```python
from build123d import *

# Parameters (mm, degrees)
SKETCH3_R                 = 2.75
BOSS_EXTRUDE3_DEPTH       = 4.5
FILLET13_R                = 15
FILLET14_START            = -4.5
FILLET14_DEPTH            = 9
SKETCH6_W                 = 69.28510074
SKETCH6_H                 = 3
CUT_EXTRUDE3_DEPTH        = 8
F_3_0MM_DOWEL_HOLE1_D     = 4
F_3_0MM_DOWEL_HOLE1_DEPTH = 9
F_3_0MM_DOWEL_HOLE1_TIP   = 1.201721238
CUT_EXTRUDE4_DEPTH        = 9
FILLET16_R                = 3
FILLET17_R                = 10
FILLET18_R                = 1.5


with BuildPart() as part:
    # Sketch3 → Boss-Extrude3 (new, symmetric)
    with BuildSketch(Plane.XY):
        with BuildLine():
            Line((0, 4), (-57, 43))
            Line((-57, 43), (-118.915266557, 43))
            ThreePointArc((-118.915266557, 43), (-123.007557158, 46.323583072), (-128.27688576, 46.488576653))
            Line((-128.27688576, 46.488576653), (-132.896667749, 45.573835187))
            ThreePointArc((-132.896667749, 45.573835187), (-135.482170861, 44.646108184), (-137.681223291, 43))
            Line((-137.681223291, 43), (-192, 43))
            Line((-192, 43), (-192, 30))
            Line((-192, 30), (-137.769349371, 30))
            Line((-137.769349371, 30), (-136.290115263, 28.079175362))
            ThreePointArc((-136.290115263, 28.079175362), (-129.185667244, 24.063000847), (-122.139231824, 28.180109937))
            Line((-122.139231824, 28.180109937), (-121.157209597, 30))
            Line((-121.157209597, 30), (-94.638255551, 30))
            Line((-94.638255551, 30), (-73.28510074, 4))
            Line((-73.28510074, 4), (-70, 4))
            Line((-70, 4), (0, 4))
        make_face()
        with BuildLine():
            Line((-124.060142597, 35.875632157), (-126.628090603, 30))
            ThreePointArc((-126.628090603, 30), (-128.04927418, 29.629254975), (-129.470457758, 30))
            Line((-129.470457758, 30), (-130.807389931, 31.612913936))
            Line((-130.807389931, 31.612913936), (-133.278796519, 34.822100799))
            ThreePointArc((-133.278796519, 34.822100799), (-133.674163723, 37.467564533), (-131.634144466, 39.197626677))
            Line((-131.634144466, 39.197626677), (-127.164353264, 40.082669168))
            ThreePointArc((-127.164353264, 40.082669168), (-124.113731215, 39.084848464), (-124.060142597, 35.875632157))
        make_face(mode=Mode.SUBTRACT)
        with Locations((-186.1, 36.5)):
            Circle(SKETCH3_R, mode=Mode.SUBTRACT)
        with Locations((-90, 36.5)):
            Circle(SKETCH3_R, mode=Mode.SUBTRACT)
    extrude(amount=BOSS_EXTRUDE3_DEPTH, both=True)

    # Fillet13
    fillet13_edges = [part.edges().sort_by_distance(p)[0] for p in [
        (-57, 43, 0),
        (-94.638255551, 30, 0),
    ]]
    fillet(fillet13_edges, radius=FILLET13_R)

    # Fillet14: read off the stored shape, not the designer's step
    # Fillet14 outline → Fillet14 (add)
    with BuildSketch(Plane.XY.offset(FILLET14_START)):
        with BuildLine():
            ThreePointArc((-122.139231824, 28.180109937), (-122.625925477, 27.42914609), (-123.191657584, 26.735774188))
            ThreePointArc((-123.191657584, 26.735774188), (-119.840432538, 29.147615588), (-115.800490823, 30))
            Line((-115.800490823, 30), (-121.157209597, 30))
            Line((-121.157209597, 30), (-122.139231824, 28.180109937))
        make_face()
        with BuildLine():
            ThreePointArc((-142.183070844, 30), (-139.084018861, 29.507674627), (-136.290115263, 28.079175362))
            Line((-136.290115263, 28.079175362), (-137.769349371, 30))
            Line((-137.769349371, 30), (-142.183070844, 30))
        make_face()
        with BuildLine():
            Line((-118.915266557, 43), (-114.686129887, 43))
            ThreePointArc((-114.686129887, 43), (-117.931187648, 43.541162856), (-120.825024465, 45.106079975))
            ThreePointArc((-120.825024465, 45.106079975), (-119.778687593, 44.13597249), (-118.915266557, 43))
        make_face()
        with BuildLine():
            ThreePointArc((-137.681223291, 43), (-136.817642976, 43.771248779), (-135.864478471, 44.428571429))
            ThreePointArc((-135.864478471, 44.428571429), (-138.342653588, 43.363758883), (-141.015266008, 43))
            Line((-141.015266008, 43), (-137.681223291, 43))
        make_face()
    extrude(amount=FILLET14_DEPTH)

    # Sketch6 → Cut-Extrude3 (cut)
    with BuildSketch(Plane.XZ.offset(-4)):
        with Locations((-34.64255037, 0)):
            Rectangle(SKETCH6_W, SKETCH6_H)
    extrude(amount=-CUT_EXTRUDE3_DEPTH, mode=Mode.SUBTRACT)

    # Ø3.0mm Dowel Hole1
    with Locations(Plane.XY.offset(4.5)):
        with Locations((-28.28510074, 8), (-58.28510074, 8)):
            Hole(F_3_0MM_DOWEL_HOLE1_D / 2, depth=F_3_0MM_DOWEL_HOLE1_DEPTH)
            with Locations((0, 0, -(F_3_0MM_DOWEL_HOLE1_DEPTH + F_3_0MM_DOWEL_HOLE1_TIP / 2))):  # 118° drill point
                Cone(0, F_3_0MM_DOWEL_HOLE1_D / 2, F_3_0MM_DOWEL_HOLE1_TIP, mode=Mode.SUBTRACT)

    # Sketch10 → Cut-Extrude4 (cut)
    with BuildSketch(Plane.XY.offset(4.5)):
        Polygon((-78.018937792, 31.515807302), (-55.600026057, 31.515807302), (-30, 14), (-63.633639909, 14), align=None)
    extrude(amount=-CUT_EXTRUDE4_DEPTH, mode=Mode.SUBTRACT)

    # Fillet16
    fillet16_edges = [part.edges().sort_by_distance(p)[0] for p in [
        (-78.018937792, 31.515807302, 0),
        (-30, 14, 0),
    ]]
    fillet(fillet16_edges, radius=FILLET16_R)

    # Fillet17
    fillet17_edges = [part.edges().sort_by_distance(p)[0] for p in [
        (-63.633639909, 14, 0),
        (-55.600026057, 31.515807302, 0),
    ]]
    fillet(fillet17_edges, radius=FILLET17_R)

    # Fillet18
    fillet18_edges = [part.edges().sort_by_distance(p)[0] for p in [
        (-192, 36.5, -4.5),
        (-192, 30, 0),
        (-192, 43, 0),
        (-192, 36.5, 4.5),
    ]]
    fillet(fillet18_edges, radius=FILLET18_R)


solid = part.part
```
For this review, take the finished solid that the model builds, in its own axes (mm). A direction names the side the tool comes from. Coordinates: 2 decimals unless noted, no trailing zeros. Loops run counter-clockwise (first coordinate to the right, second up) from the corner with the lowest first, then second, coordinate; pieces in that order, holes last.
1. Add section C-C, the plane x = -19.5. Give the boundary of the cut face in (y, z), then the cut area to 3 significant figures.
2. For line 1 (Y direction, x = -186.1, z = -1); line 2 (X direction, y = 26.5, z = 4); line 3 (X direction, y = 8, z = -2.2), list the stretches that pass through material, from the lowest coordinate up.
3. Add section D-D, the plane x = -144. Give the boundary of the cut face in (y, z).
4. Insertion check: P1, Ø4.5, axis at x = -155, z = -1, coming from the -Y side; P2, Ø5, axis at x = -58.29, y = 8, coming from the -Z side; P3, Ø1.5, axis at y = 30, z = 3.5, coming from the -X side; P4, Ø3, axis at x = -28.29, y = 8, coming from the -Z side. Each pin has a flat end and moves straight along its axis. Give the tip position at first contact, or say it passes through.
5. Mouldability with a two-part tool opening along Z and no side actions: class faces 1 (the flat face through (-69.285, 8, 0)), 2 (the flat face through (-165, 43, 0)), 3 (the flat face through (-97, 30, -4.5)) as +Z half, -Z half, draft (parallel to the pull), parting line (faces both ways), or undercut.
6. Add section B-B, the plane y = 8. Give the boundary of the cut face in (x, z).
7. For faces 4 (the cylindrical face through (-119.894, 29.124, -0.063)), 5 (the flat face through (-37, 4, 2)), 6 (the flat face through (-88, 43, 0)), 7 (the flat face through (-130.55, 46.04, 0.06)), 8 (the cylindrical face through (-63.24, 14.99, -0.06)), list the 3-axis set-ups (+Z, -Z, +X, -X, +Y, -Y) from which the entire face can be reached by the end or side of a thin tool; tool diameter is ignored.
8. Add section A-A, the plane x = -186.1. Give the boundary of the cut face in (y, z), then the cut area to 3 significant figures.
Result:
1. outline: (4, -4.5) - (17.34, -4.5) - (17.34, 4.5) - (4, 4.5) - (4, 1.5) - (12, 1.5) - (12, -1.5) - (4, -1.5) - close
1. area: 96.1 mm2
2. line 1: y = 30 to 33.75, 39.25 to 43
2. line 2: x = -135.07 to -123.42, -92.1 to -73.9, -48.27 to -32.88
2. line 3: x = -76.57 to -60.29, -56.29 to -30.29, -26.29 to -5.85
3. outline: (30, -4.5) - (43, -4.5) - (43, 4.5) - (30, 4.5) - close
4. P1: stops at y = 30
4. P2: stops at z = -4.5
4. P3: stops at x = -191.8
4. P4: passes through
5. face 1: undercut
5. face 2: draft
5. face 3: -Z half
6. outline: (-76.57, -4.5) - (-60.29, -4.5) - (-60.29, -1.5) - (-69.29, -1.5) - (-69.29, 1.5) - (-60.29, 1.5) - (-60.29, 4.5) - (-76.57, 4.5) - close; (-56.29, -4.5) - (-30.29, -4.5) - (-30.29, -1.5) - (-56.29, -1.5) - close; (-56.29, 1.5) - (-30.29, 1.5) - (-30.29, 4.5) - (-56.29, 4.5) - close; (-26.29, -4.5) - (-5.85, -4.5) - (-5.85, -1.5) - (-26.29, -1.5) - close; (-26.29, 1.5) - (-5.85, 1.5) - (-5.85, 4.5) - (-26.29, 4.5) - close
7. face 4: +Z, -Z, -Y
7. face 5: +Z, -Z, +X, -X, -Y
7. face 6: +Z, -Z, +X, +Y
7. face 7: +Z, -Z, -X, +Y
7. face 8: +Z, -Z
8. outline: (30, -4.5) - (33.75, -4.5) - (33.75, 4.5) - (30, 4.5) - close; (39.25, -4.5) - (43, -4.5) - (43, 4.5) - (39.25, 4.5) - close
8. area: 67.5 mm2
